Build history of the part. All positions in model axes, mm. A direction names the side the tool comes from. Round coordinates to 2 decimals unless told otherwise and drop trailing zeros. Write each loop counter-clockwise with the first axis right and the second up, starting at its lowest first coordinate (ties: lowest second). Pieces come first, ordered by that corner, then holes. Notation, with made-up numbers: M 11.25,76 L 62.25,76 A23 ccw 62.25,97 Z; hole C 76,-31.5 d11. An arc over 180 degrees is marked long. Use a Markdown table: item, result.
from build123d import *

# Parameters (mm, degrees)
SKETCH1_W           = 6
SKETCH1_H           = 6
SKETCH1_R           = 2.5
SKETCH1_R_2         = 1.55
BOSS_EXTRUDE1_DEPTH = 3
SKETCH1_3_R         = 1.55
BOSS_EXTRUDE2_DEPTH = 3
SKETCH1_4_R         = 2.5
SKETCH1_4_R_2       = 1.55
BOSS_EXTRUDE3_DEPTH = 20


with BuildPart() as part:
    # Sketch1 → Boss-Extrude1 (new body)
    with BuildSketch(Plane(origin=(0, 0, 0), x_dir=(1, 0, 0), z_dir=(0, 1, 0))):
        Rectangle(SKETCH1_W, SKETCH1_H)
        Circle(SKETCH1_R, mode=Mode.SUBTRACT)
        Circle(SKETCH1_R)
        Circle(SKETCH1_R_2, mode=Mode.SUBTRACT)
        Circle(SKETCH1_R_2)
    extrude(amount=-BOSS_EXTRUDE1_DEPTH)

    # Sketch1_3 → Boss-Extrude2 (add)
    with BuildSketch(Plane(origin=(0, 0, 0), x_dir=(1, 0, 0), z_dir=(0, 1, 0))):
        Circle(SKETCH1_3_R)
    extrude(amount=BOSS_EXTRUDE2_DEPTH)

    # Sketch1_4 → Boss-Extrude3 (add)
    with BuildSketch(Plane(origin=(0, 0, 0), x_dir=(1, 0, 0), z_dir=(0, 1, 0))):
        Circle(SKETCH1_4_R)
        Circle(SKETCH1_4_R_2, mode=Mode.SUBTRACT)
    extrude(amount=BOSS_EXTRUDE3_DEPTH)


solid = part.part
Q1. Cut at D-D on z = 0. Give the cut face in (x, y), and give its area (3 significant figures).
Response values:
| item | result |
|---|---|
| outline | M -3,-3 L 3,-3 L 3,0 L 2.5,0 L 2.5,20 L 1.55,20 L 1.55,3 L -1.55,3 L -1.55,20 L -2.5,20 L -2.5,0 L -3,0 Z |
| area | 65.3 mm2 |
Q2. Cut at A-A on x = 0. Give the cut face in (y, z).
Response values:
| item | result |
|---|---|
| outline | M -3,-3 L 0,-3 L 0,-2.5 L 20,-2.5 L 20,-1.55 L 3,-1.55 L 3,1.55 L 20,1.55 L 20,2.5 L 0,2.5 L 0,3 L -3,3 Z |
Q3. Drill centre lines: L1, parallel to X at y = 12.25, z = 0; L2, parallel to Y at x = -2.6, z = 1.45. Where is each one in solid material? Low to high.
Response values:
| item | result |
|---|---|
| L1 | x = -2.5 to -1.55, 1.55 to 2.5 |
| L2 | y = -3 to 0 |
Q4. Cut at C-C on y = 18.75. Give the cut face in (x, z), and give its area (3 significant figures).
Response values:
| item | result |
|---|---|
| outline | C 0,0 d5; hole C 0,0 d3.1 |
| area | 12.1 mm2 |
Q5. Two-plate mould, pull along Z, no slides. Class faces 1 (the flat face through (0, -1, -3)), 2 (the cylindrical face through (0.715, 11.381, 1.375)), 3 (the flat face through (0, -3, 0)): +Z half, -Z half, draft (parallel to the pull), parting line (faces both ways), or undercut.
Response values:
| item | result |
|---|---|
| face 1 | -Z half |
| face 2 | undercut |
| face 3 | draft |
Q6. Cut at B-B on z = 2.2. Give the cut face in (x, y), and give its area (3 significant figures).
Response values:
| item | result |
|---|---|
| outline | M -3,-3 L 3,-3 L 3,0 L 1.19,0 L 1.19,20 L -1.19,20 L -1.19,0 L -3,0 Z |
| area | 65.5 mm2 |
Q7. Drop flat-ended pins along their axis: P1, Ø1.5, axis at x = -1, y = 14, coming from the +Z side; P2, Ø3, axis at y = 3, z = -1.5, coming from the -X side. Give the stop position or say it passes through.
Response values:
| item | result |
|---|---|
| P1 | stops at z = 2.49 |
| P2 | stops at x = -2.5 |
Q8. Which spindle directions (+Z, -Z, +X, -X, +Y, -Y) get a long thin tool onto all of the face, cutting with end or side? Do faces 4 (the flat face through (0, -1, 3)), 5 (the flat face through (-2.7, 0, 0)). Say none if no direction does.
Response values:
| item | result |
|---|---|
| face 4 | +Z, +X, -X, +Y, -Y |
| face 5 | +Y |
